Geometry check sheet. Reference: the model listing, model coordinates, mm. Coordinates: 2 decimals unless noted, no trailing zeros. Write each loop counter-clockwise with the first axis right and the second up, starting at its lowest first coordinate (ties: lowest second). Pieces come first, ordered by that corner, then holes. Notation, with made-up numbers: (88, 44) -> (121, 44) arc R20 ccw to (121, 69) -> close; hole circle Ø1 at (-18, 69.5). An arc over 180 degrees is marked (long way). Use a Markdown table: item, result.
```python
from build123d import *

# Parameters (mm, degrees)
SKETCH2_R           = 14
BOSS_EXTRUDE1_DEPTH = 23
SKETCH3_R           = 6.05
CUT_EXTRUDE1_DEPTH  = 31.347981811
CHAMFER1_SIZE       = 0.5


with BuildPart() as part:
    # Sketch2 → Boss-Extrude1 (new body)
    with BuildSketch(Plane(origin=(0, 0, 0), x_dir=(1, 0, 0), z_dir=(0, 1, 0))):
        with Locations(Location((0, 0, 0), (0, 0, 270))):
            Circle(SKETCH2_R)
    extrude(amount=BOSS_EXTRUDE1_DEPTH)

    # Sketch3 → Cut-Extrude1 (cut, through all)
    with BuildSketch(Plane(origin=(0, 23, 0), x_dir=(1, 0, 0), z_dir=(0, 1, 0))):
        with Locations(Location((0, 0, 0), (0, 0, 270))):
            Circle(SKETCH3_R)
    extrude(amount=-CUT_EXTRUDE1_DEPTH, mode=Mode.SUBTRACT)

    # Chamfer1
    chamfer1_edges = [part.edges().sort_by_distance(p)[0] for p in [
        (0, 0, -14),
        (0, 23, -14),
    ]]
    chamfer(chamfer1_edges, length=CHAMFER1_SIZE)


solid = part.part
```
Item 1: Section check B-B on z = 0. Record the boundary of the cut face in (x, y), then the cut area to 3 significant figures.
Answer block:
| item | result |
|---|---|
| outline | (-14, 0.5) -> (-13.5, 0) -> (-6.05, 0) -> (-6.05, 23) -> (-13.5, 23) -> (-14, 22.5) -> close; (6.05, 0) -> (13.5, 0) -> (14, 0.5) -> (14, 22.5) -> (13.5, 23) -> (6.05, 23) -> close |
| area | 365 mm^2 |
Item 2: Section check A-A on x = 0. Record the boundary of the cut face in (y, z), then the cut area to 3 significant figures.
Answer block:
| item | result |
|---|---|
| outline | (0, -13.5) -> (0.5, -14) -> (22.5, -14) -> (23, -13.5) -> (23, -6.05) -> (0, -6.05) -> close; (0, 6.05) -> (23, 6.05) -> (23, 13.5) -> (22.5, 14) -> (0.5, 14) -> (0, 13.5) -> close |
| area | 365 mm^2 |
Item 3: Mould release check, pull along X, two halves, no side actions. Record for faces 1 (the flat face through (-3, 23, 6)), 2 (the cylindrical face through (-13.67, 11.35, -3.03)), 3 (the cylindrical face through (1.82, 11.66, 5.77)): +X half, -X half, draft (parallel to the pull), parting line (faces both ways), or undercut.
Answer block:
| item | result |
|---|---|
| face 1 | draft |
| face 2 | parting line |
| face 3 | undercut |
Item 4: Depth check by flat-ended pin: P1, Ø10, axis at x = 7.5, y = 20.5, coming from the -Z side (3 decimals); P2, Ø10, axis at y = 3.5, z = 10.5, coming from the +X side; P3, Ø4, axis at y = 13.5, z = -8, coming from the +X side. Enter the tip coordinate at first touch or a pass-through.
Answer block:
| item | result |
|---|---|
| P1 | stops at z = -13.775 |
| P2 | stops at x = 12.87 |
| P3 | stops at x = 12.65 |
Item 5: Thickness scan on L1, parallel to X at y = 9.25, z = 0; L2, parallel to X at y = 9.5, z = 3.5; L3, parallel to Z at x = -5.5, y = 1.25. Record the ranges inside material, lowest first. Write a range as [from, to].
Answer block:
| item | result |
|---|---|
| L1 | x = [-14, -6.05], [6.05, 14] |
| L2 | x = [-13.56, -4.93], [4.93, 13.56] |
| L3 | z = [-12.87, -2.52], [2.52, 12.87] |
Item 6: Section check C-C on y = 1.5. Record the boundary of the cut face in (x, z).
Answer block:
| item | result |
|---|---|
| outline | circle Ø28 at (0, 0); hole circle Ø12.1 at (0, 0) |
